The model under review builds one solid part; all positions refer to its coordinate system, in mm. Face numbers are marked on the shaded views. Round coordinates to 2 decimals unless told otherwise and drop trailing zeros. Order: outer loops, then holes, each group sorted by start corner. A loop starts at its lowest first (then second) coordinate and runs counter-clockwise, first axis right, second up.
from build123d import *

# Parameters (mm, degrees)
SKETCH4_R           = 68
SKETCH4_R_2         = 2.5
BOSS_EXTRUDE5_DEPTH = 3
SKETCH5_R           = 71
SKETCH5_R_2         = 68
BOSS_EXTRUDE6_DEPTH = 40


with BuildPart() as part:
    # Sketch4 → Boss-Extrude5 (new body)
    with BuildSketch(Plane(origin=(0, 0, 0), x_dir=(1, 0, 0), z_dir=(0, 1, 0))):
        with BuildLine():
            Line((-71.5, 74.5), (71.5, 74.5))
            ThreePointArc((71.5, 74.5), (73.621320344, 73.621320344), (74.5, 71.5))
            Line((74.5, 71.5), (74.5, -71.5))
            ThreePointArc((74.5, -71.5), (73.621320344, -73.621320344), (71.5, -74.5))
            Line((71.5, -74.5), (-71.5, -74.5))
            ThreePointArc((-71.5, -74.5), (-73.621320344, -73.621320344), (-74.5, -71.5))
            Line((-74.5, -71.5), (-74.5, 71.5))
            ThreePointArc((-74.5, 71.5), (-73.621320344, 73.621320344), (-71.5, 74.5))
        make_face()
        Circle(SKETCH4_R, mode=Mode.SUBTRACT)
        with Locations((-62.5, 62.5)):
            Circle(SKETCH4_R_2, mode=Mode.SUBTRACT)
        with Locations((62.5, 62.5)):
            Circle(SKETCH4_R_2, mode=Mode.SUBTRACT)
        with Locations((62.5, -62.5)):
            Circle(SKETCH4_R_2, mode=Mode.SUBTRACT)
        with Locations((-62.5, -62.5)):
            Circle(SKETCH4_R_2, mode=Mode.SUBTRACT)
    extrude(amount=BOSS_EXTRUDE5_DEPTH)

    # Sketch5 → Boss-Extrude6 (add)
    with BuildSketch(Plane(origin=(0, 3, 0), x_dir=(1, 0, 0), z_dir=(0, 1, 0))):
        Circle(SKETCH5_R)
        Circle(SKETCH5_R_2, mode=Mode.SUBTRACT)
    extrude(amount=BOSS_EXTRUDE6_DEPTH)


solid = part.part
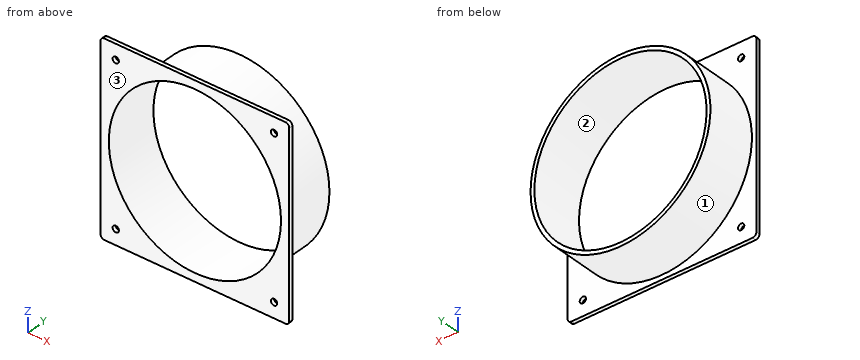
(1) The part is to be moulded in two halves that separate along X. For the marked faces 1, 2 and 3, say which applies: pulls with the +X half, pulls with the -X half, needs draft (parallel to the pull), parting line crosses it, or undercut.
(2) To check wall thickness, follow L1, parallel to X at y = 1.9, z = 62.5; L2, parallel to X at y = 27, z = 0. State the ranges of each line that lie inside material, in increasing order.
(3) We need section B-B (x = 0). Give the boundary of the cut face in (y, z).
(4) We need section A-A (z = -26.5). Give the boundary of the cut face in (x, y), and give its area (3 significant figures).
(5) We need section D-D (y = 7). Give the boundary of the cut face in (x, z).
(6) Clearance check with flat-ended pins moving along their axes: P1, Ø8, axis at x = -62.5, z = 62.5, coming from the -Y side; P2, Ø3, axis at y = 28, z = -3.5, coming from the -X side; P3, Ø2, axis at y = 23.5, z = 28, coming from the -X side; P4, Ø3, axis at x = 59, y = 34, coming from the -Z side. State where each tip first meets the part, or that it passes through.
(7) We need section C-C (x = -62.5). Give the boundary of the cut face in (y, z).
Verdict:
1. face 1: parting line crosses it
1. face 2: undercut
1. face 3: needs draft
2. L1: x = -74.5 to -65, -60 to -26.79, 26.79 to 60, 65 to 74.5
2. L2: x = -71 to -68, 68 to 71
3. outline: (0, -74.5) - (3, -74.5) - (3, -71) - (43, -71) - (43, -68) - (0, -68) - close; (0, 68) - (43, 68) - (43, 71) - (3, 71) - (3, 74.5) - (0, 74.5) - close
4. outline: (-74.5, 0) - (-62.62, 0) - (-62.62, 43) - (-65.87, 43) - (-65.87, 3) - (-74.5, 3) - close; (62.62, 0) - (74.5, 0) - (74.5, 3) - (65.87, 3) - (65.87, 43) - (62.62, 43) - close
4. area: 331 mm2
5. outline: circle Ø142 at (0, 0); hole circle Ø136 at (0, 0)
6. P1: stops at y = 0
6. P2: stops at x = -70.97
6. P3: stops at x = -65.67
6. P4: stops at z = -41.65
7. outline: (0, -74.5) - (3, -74.5) - (3, -65) - (0, -65) - close; (0, -60) - (3, -60) - (3, -33.69) - (43, -33.69) - (43, -26.79) - (0, -26.79) - close; (0, 26.79) - (43, 26.79) - (43, 33.69) - (3, 33.69) - (3, 60) - (0, 60) - close; (0, 65) - (3, 65) - (3, 74.5) - (0, 74.5) - close
